Geometry check sheet. Reference: the model listing, model coordinates, mm. A direction names the side the tool comes from. Give positions to 0.01 mm unless a question says otherwise; leave off trailing zeros. Write each loop counter-clockwise with the first axis right and the second up, starting at its lowest first coordinate (ties: lowest second). Pieces come first, ordered by that corner, then holes. Notation, with made-up numbers: (51, 52.5) - (106, 52.5) arc R34 ccw to (106, 84.5) - close; hole circle Ø4 at (42, 89). An arc over 180 degrees is marked (long way). Use a Markdown table: item, result.
```python
from build123d import *
from build123d.topology import SkipClean

# Parameters (mm, degrees)
SKETCH1_W               = 60
SKETCH1_H               = 60
BOSS_EXTRUDE1_DEPTH     = 90
CUT_EXTRUDE1_DEPTH      = 100.498743711
CUT_EXTRUDE1_DEPTH_BACK = 100.498743711
SKETCH2_W               = 40.7
SKETCH2_H               = 26
SKETCH4_W               = 36
SKETCH4_H               = 38
CUT_EXTRUDE2_DEPTH      = 113.249721603
SKETCH5_W               = 36
SKETCH5_H               = 34
CUT_EXTRUDE3_DEPTH      = 79
SKETCH6_R               = 19.5
CUT_EXTRUDE4_DEPTH      = 20
FILLET2_R               = 6
FILLET3_START           = -30
FILLET3_DEPTH           = 60
FILLET3_2_DEPTH         = 13
FILLET3_START_2         = 17
FILLET3_3_DEPTH         = 13
CHAMFER1_SIZE           = 3
SKETCH7_R               = 3.05
CUT_EXTRUDE5_DEPTH      = 104.230276693
SKETCH8_R               = 5.4
CUT_EXTRUDE6_DEPTH      = 9.5
CHAMFER2_SIZE           = 1
SKETCH10_R              = 2.4
CUT_EXTRUDE7_DEPTH      = 23
CHAMFER3_SIZE           = 3
SKETCH11_R              = 4
CUT_EXTRUDE8_DEPTH      = 40
SKETCH12_R              = 2
CUT_EXTRUDE9_DEPTH      = 11


with BuildPart() as part:
    # Sketch1 → Boss-Extrude1 (new body)
    with BuildSketch(Plane(origin=(0, 0, 0), x_dir=(1, 0, 0), z_dir=(0, 1, 0))):
        Rectangle(SKETCH1_W, SKETCH1_H)
    extrude(amount=BOSS_EXTRUDE1_DEPTH)

    # Sketch2 → Cut-Extrude1 (cut, two sides: drawn at the far end of the back side and taken through both)
    with BuildSketch(Plane(origin=(0, 0, 0), x_dir=(0, 0, -1), z_dir=(1, 0, 0)).offset(-CUT_EXTRUDE1_DEPTH_BACK)):
        with Locations((9.65, 13)):
            Rectangle(SKETCH2_W, SKETCH2_H)
    extrude(amount=CUT_EXTRUDE1_DEPTH + CUT_EXTRUDE1_DEPTH_BACK, mode=Mode.SUBTRACT)

    # Sketch4 → Cut-Extrude2 (cut, through all)
    with BuildSketch(Plane(origin=(0, 0, -30), x_dir=(-1, 0, 0), z_dir=(0, 0, -1))):
        with Locations((0, 60)):
            Rectangle(SKETCH4_W, SKETCH4_H)
    extrude(amount=-CUT_EXTRUDE2_DEPTH, mode=Mode.SUBTRACT)

    # Sketch5 → Cut-Extrude3 (cut)
    with BuildSketch(Plane.XZ):
        Rectangle(SKETCH5_W, SKETCH5_H)
    extrude(amount=-CUT_EXTRUDE3_DEPTH, mode=Mode.SUBTRACT)

    # Sketch6 → Cut-Extrude4 (cut)
    with BuildSketch(Plane(origin=(0, 90, 0), x_dir=(1, 0, 0), z_dir=(0, 1, 0))):
        with Locations(Location((0, 0, 0), (0, 0, 270))):
            Circle(SKETCH6_R)
    extrude(amount=-CUT_EXTRUDE4_DEPTH, mode=Mode.SUBTRACT)

    # Fillet2
    # the kernel refuses this fillet: 6 mm, written as the material it adds along each edge
    with BuildSketch(Plane(origin=(0, 70, 0), x_dir=(-0.39557733724118155, 0, -0.9184326705105695), z_dir=(0.9184326705105695, 0, -0.39557733724118155))) as fillet2_piece_1_section:
        with BuildLine():
            CenterArc((19.5 - FILLET2_R, FILLET2_R), FILLET2_R, 270, 90)
            Line((19.5 - FILLET2_R, 0), (19.5, 0))
            Line((19.5, 0), (19.5, FILLET2_R))
        make_face()
    fillet2_piece_1 = revolve(axis=Axis((0, 70, 0), (0, 1, 0)), revolution_arc=133.396028061, mode=Mode.PRIVATE)
    fillet2_piece_1 = split(fillet2_piece_1, bisect_by=Plane(origin=(-18, 70, 0), z_dir=(-1, 0, 0)), keep=Keep.TOP, mode=Mode.PRIVATE)
    add(fillet2_piece_1)
    with BuildSketch(Plane(origin=(0, 70, 0), x_dir=(0.39557733724118166, 0, 0.9184326705105695), z_dir=(-0.9184326705105695, 0, 0.39557733724118166))) as fillet2_piece_2_section:
        with BuildLine():
            CenterArc((19.5 - FILLET2_R, FILLET2_R), FILLET2_R, 270, 90)
            Line((19.5 - FILLET2_R, 0), (19.5, 0))
            Line((19.5, 0), (19.5, FILLET2_R))
        make_face()
    fillet2_piece_2 = revolve(axis=Axis((0, 70, 0), (0, 1, 0)), revolution_arc=133.396028061, mode=Mode.PRIVATE)
    fillet2_piece_2 = split(fillet2_piece_2, bisect_by=Plane(origin=(18, 70, 0), z_dir=(1, 0, 0)), keep=Keep.TOP, mode=Mode.PRIVATE)
    add(fillet2_piece_2)

    # Fillet3: read off the stored shape, not the designer's step
    # Fillet3 outline → Fillet3 (add)
    with BuildSketch(Plane.XY.offset(FILLET3_START)):
        with BuildLine():
            ThreePointArc((-18, 70), (-15.363961031, 76.363961031), (-9, 79))
            Line((-9, 79), (-18, 79))
            Line((-18, 79), (-18, 70))
        make_face()
        with BuildLine():
            Line((18, 79), (9, 79))
            ThreePointArc((9, 79), (15.363961031, 76.363961031), (18, 70))
            Line((18, 70), (18, 79))
        make_face()
    extrude(amount=FILLET3_DEPTH)

    # Fillet3 2 outline → Fillet3 2 (add)
    with BuildSketch(Plane.XY.offset(FILLET3_START)):
        with BuildLine():
            ThreePointArc((-9, 41), (-15.363961031, 43.636038969), (-18, 50))
            Line((-18, 50), (-18, 41))
            Line((-18, 41), (-9, 41))
        make_face()
        with BuildLine():
            Line((18, 41), (18, 50))
            ThreePointArc((18, 50), (15.363961031, 43.636038969), (9, 41))
            Line((9, 41), (18, 41))
        make_face()
    extrude(amount=FILLET3_2_DEPTH)

    # Fillet3 3 outline → Fillet3 3 (add)
    with BuildSketch(Plane.XY.offset(FILLET3_START_2)):
        with BuildLine():
            ThreePointArc((-9, 41), (-15.363961031, 43.636038969), (-18, 50))
            Line((-18, 50), (-18, 41))
            Line((-18, 41), (-9, 41))
        make_face()
        with BuildLine():
            Line((18, 41), (18, 50))
            ThreePointArc((18, 50), (15.363961031, 43.636038969), (9, 41))
            Line((9, 41), (18, 41))
        make_face()
    extrude(amount=FILLET3_3_DEPTH)

    # Fillet3 4 outline → Fillet3 4 (revolve, cut)
    with SkipClean():  # the faces are left unmerged after this step: merging them gives an invalid solid
        with BuildSketch(Plane.XY):
            with BuildLine():
                Line((0, 71.827932396), (17.812058894, 71.827932396))
                ThreePointArc((17.812058894, 71.827932396), (19.062029907, 73.749705949), (19.5, 76))
                Line((19.5, 76), (19.5, 79))
                Line((19.5, 79), (0, 79))
                Line((0, 79), (0, 71.827932396))
            make_face()
        revolve(axis=Axis((0, 0, 0), (0, 1, 0)), mode=Mode.SUBTRACT)
    add(part.part.scale(1), mode=Mode.REPLACE)  # the faces are merged on a copy

    # Chamfer1
    chamfer1_edges = [part.edges().sort_by_distance(p)[0] for p in [
        (-30, 58, -30),
        (30, 58, -30),
        (30, 45, 30),
        (-30, 45, 30),
    ]]
    chamfer(chamfer1_edges, length=CHAMFER1_SIZE)

    # Sketch7 → Cut-Extrude5 (cut, through all)
    with BuildSketch(Plane(origin=(0, 0, 10.7), x_dir=(-1, 0, 0), z_dir=(0, 0, -1))):
        with Locations((-23, 20)):
            Circle(SKETCH7_R)
        with Locations((-23, 7)):
            Circle(SKETCH7_R)
        with Locations((23, 20)):
            Circle(SKETCH7_R)
        with Locations((23, 7)):
            Circle(SKETCH7_R)
    extrude(amount=-CUT_EXTRUDE5_DEPTH, mode=Mode.SUBTRACT)

    # Sketch8 → Cut-Extrude6 (cut)
    with BuildSketch(Plane.XY.offset(30)):
        with Locations((-23, 20)):
            Circle(SKETCH8_R)
        with Locations((23, 20)):
            Circle(SKETCH8_R)
        with Locations((23, 7)):
            Circle(SKETCH8_R)
        with Locations((-23, 7)):
            Circle(SKETCH8_R)
    extrude(amount=-CUT_EXTRUDE6_DEPTH, mode=Mode.SUBTRACT)

    # Chamfer2
    chamfer2_edges = [part.edges().sort_by_distance(p)[0] for p in [
        (-30, 0, 18.85),
        (-30, 26, -8.15),
        (0, 26, -30),
        (30, 26, -8.15),
        (28.5, 26, -28.5),
        (-28.5, 26, -28.5),
        (30, 0, 18.85),
        (0, 0, 30),
        (28.5, 0, 28.5),
        (-28.5, 0, 28.5),
        (-24, 0, 10.7),
        (-30, 13, 10.7),
        (30, 13, 10.7),
        (24, 0, 10.7),
        (-18, 0, 13.85),
        (18, 0, 13.85),
        (0, 0, 17),
    ]]
    chamfer(chamfer2_edges, length=CHAMFER2_SIZE)

    # Sketch10 → Cut-Extrude7 (cut)
    with BuildSketch(Plane(origin=(0, 90, 0), x_dir=(1, 0, 0), z_dir=(0, 1, 0))):
        with Locations(Location((-23.59, 23.59, 0), (0, 0, 270))):
            Circle(SKETCH10_R)
        with Locations(Location((23.59, 23.59, 0), (0, 0, 270))):
            Circle(SKETCH10_R)
        with Locations(Location((23.59, -23.59, 0), (0, 0, 270))):
            Circle(SKETCH10_R)
        with Locations(Location((-23.59, -23.59, 0), (0, 0, 270))):
            Circle(SKETCH10_R)
    extrude(amount=-CUT_EXTRUDE7_DEPTH, mode=Mode.SUBTRACT)

    # Chamfer3
    chamfer3_edges = [part.edges().sort_by_distance(p)[0] for p in [
        (-18, 60, 30),
        (-18, 60, -30),
        (0, 79, 30),
        (18, 60, -30),
        (18, 60, 30),
        (0, 41, 30),
        (0, 41, -30),
        (-15.363961031, 76.363961031, -30),
        (-15.363961031, 76.363961031, 30),
        (15.363961031, 76.363961031, -30),
        (15.363961031, 76.363961031, 30),
        (15.363961031, 43.636038969, 30),
        (15.363961031, 43.636038969, -30),
        (-15.363961031, 43.636038969, -30),
        (-15.363961031, 43.636038969, 30),
        (0, 79, -30),
    ]]
    chamfer(chamfer3_edges, length=CHAMFER3_SIZE)

    # Sketch11 → Cut-Extrude8 (cut)
    with BuildSketch(Plane.XZ):
        with Locations(Location((0, 22.24, 0), (0, 0, 270))):
            Circle(SKETCH11_R)
    extrude(amount=-CUT_EXTRUDE8_DEPTH, mode=Mode.SUBTRACT)

    # Sketch12 → Cut-Extrude9 (cut)
    with BuildSketch(Plane.XZ):
        with Locations(Location((-12, 22.24, 0), (0, 0, 270))):
            Circle(SKETCH12_R)
        with Locations(Location((12, 22.24, 0), (0, 0, 270))):
            Circle(SKETCH12_R)
    extrude(amount=-CUT_EXTRUDE9_DEPTH, mode=Mode.SUBTRACT)


solid = part.part
```
1) Set-up check for faces 4 (the conical face through (16.04, 43.11, -27.85)), 5 (the cylindrical face through (-15.294, 43.566, 21.93)), 6 (the flat face through (-19, 60, 28)): record each of +Z, -Z, +X, -X, +Y, -Y from which the full face is reachable in a straight line by a thin tool's end or side.
Working result:
| item | result |
|---|---|
| face 4 | -Z |
| face 5 | +Z, -Z |
| face 6 | +Z |
2) Section check A-A on x = 0. Record the boundary of the cut face in (y, z).
Working result:
| item | result |
|---|---|
| outline | (0, 18) - (1, 17) - (41, 17) - (41, 27) - (38, 30) - (1, 30) - (0, 29) - (0, 26.24) - (40, 26.24) - (40, 18.24) - (0, 18.24) - close; (26, -29) - (27, -30) - (38, -30) - (41, -27) - (41, -17) - (26, -17) - close; (79, -27) - (82, -30) - (90, -30) - (90, -19.5) - (79, -19.5) - close; (79, 19.5) - (90, 19.5) - (90, 30) - (82, 30) - (79, 27) - close |
3) Section check D-D on x = 23.59. Count the separate pieces of the cut face and the enclosed holes in it, then the cut area to 3 significant figures.
Working result:
| item | result |
|---|---|
| separate pieces | 3 |
| enclosed holes | 0 |
| area | 3,800 mm² |
4) Mould release check, pull along Z, two halves, no side actions. Record for faces 1 (the flat face through (24, 67, 24)), 2 (the flat face through (0, 80, 28)), 3 (the cylindrical face through (15.434, 43.706, 21.93)): pulls with the +Z half, pulls with the -Z half, needs draft (parallel to the pull), parting line crosses it, or undercut.
Working result:
| item | result |
|---|---|
| face 1 | undercut |
| face 2 | pulls with the +Z half |
| face 3 | needs draft |
5) Depth check by flat-ended pin: P1, Ø6.5, axis at x = 23, y = 20, coming from the +Z side; P2, Ø5.5, axis at x = -21.5, y = 12.5, coming from the -Z side; P3, Ø10, axis at x = -15, z = -15.5, coming from the -Y side. Enter the tip coordinate at first touch or a pass-through.
Working result:
| item | result |
|---|---|
| P1 | stops at z = 20.5 |
| P2 | stops at z = 10.7 |
| P3 | stops at y = 26 |
6) Section check C-C on z = -23.59. Record the boundary of the cut face in (x, y).
Working result:
| item | result |
|---|---|
| outline | (-30, 27) - (-29, 26) - (29, 26) - (30, 27) - (30, 90) - (25.99, 90) - (25.99, 67) - (21.19, 67) - (21.19, 90) - (-21.19, 90) - (-21.19, 67) - (-25.99, 67) - (-25.99, 90) - (-30, 90) - close; hole (-18, 50) arc R9 ccw to (-9, 41) - (9, 41) arc R9 ccw to (18, 50) - (18, 70) arc R9 ccw to (9, 79) - (-9, 79) arc R9 ccw to (-18, 70) - close |
7) Section check B-B on z = 15. Record the boundary of the cut face in (x, y), then the cut area to 3 significant figures.
Working result:
| item | result |
|---|---|
| outline | (-30, 1) - (-29, 0) - (-19, 0) - (-18, 1) - (-18, 70) arc R9 cw to (-12.46, 78.31) - (-12.46, 90) - (-30, 90) - close; (12.46, 78.31) arc R9 cw to (18, 70) - (18, 1) - (19, 0) - (29, 0) - (30, 1) - (30, 90) - (12.46, 90) - close; hole circle Ø6.1 at (-23, 7); hole circle Ø6.1 at (-23, 20); hole circle Ø6.1 at (23, 7); hole circle Ø6.1 at (23, 20) |
| area | 2,200 mm² |
8) Material ranges on L1, parallel to Y at x = 23, z = 15.25; L2, parallel to Y at x = -23, z = 25.5; L3, parallel to X at y = 12, z = 22, recorded low to high. Write a range as from..to.
Working result:
| item | result |
|---|---|
| L1 | y = 0..3.95, 10.05..16.95, 23.05..90 |
| L2 | y = 0..1.6, 12.4..14.6, 25.4..67 |
| L3 | x = -30..-25.04, -20.96..-3.99, 3.99..20.96, 25.04..30 |
